Design review of the part shown in the three views and the two pictorial views. Dimensions are in mm from the part's minimum x, y and z. A direction names the side the tool comes from. Round coordinates to 2 decimals unless told otherwise and drop trailing zeros. Order: outer loops, then holes, each group sorted by start corner. A loop starts at its lowest first (then second) coordinate and runs counter-clockwise, first axis right, second up. Notation, with made-up numbers: (18, 72) - (72, 72) arc R4 ccw to (72, 77) - close; hole circle Ø11 at (35.5, -17.5). An arc over 180 degrees is marked (long way). One line per question, with ' | ' between items. Start each with the question number.
Item 1: Tool access review of the marked faces 4, 5, 6 and 7: name each direction out of +Z, -Z, +X, -X, +Y, -Y from which nothing blocks a thin tool from reaching the whole face with its end or side.
Item 2: Add section A-A on y = 6.35. State the section outline as (x, z) points, and give its area (3 significant figures).
Item 3: Draft analysis for pull direction X (two halves, no side actions). For the marked faces 1, 2 and 3, state which applies: +X half, -X half, draft (parallel to the pull), parting line (faces both ways), or undercut.
Item 4: Add section D-D on y = 10.5. State the section outline as (x, z) points.
Item 5: For L1, parallel to X at y = 14.85, z = 19; L2, parallel to Y at x = 5, z = 8; L3, parallel to X at y = 15.1, z = 9, list the stretches that pass through material, from the lowest coordinate up. Write a range as [from, to].
Item 6: Insertion check: pin 1 Ø1 at (y, z) = (13, 14.5) entering from -X; pin 2 Ø8 at (x, z) = (30.5, 22) entering from -Y; pin 3 Ø4 at (y, z) = (1.5, 12.5) entering from +X; pin 4 Ø6 at (x, y) = (52, 14.5) entering from +Z. Each pin has a flat end and moves straight along its axis. Give the tip position at first contact, or say it passes through.
Item 7: Add section C-C on z = 8. State the section outline as (x, y) points.
Item 8: Add section B-B on x = 55. State the section outline as (y, z) points, and give its area (3 significant figures).
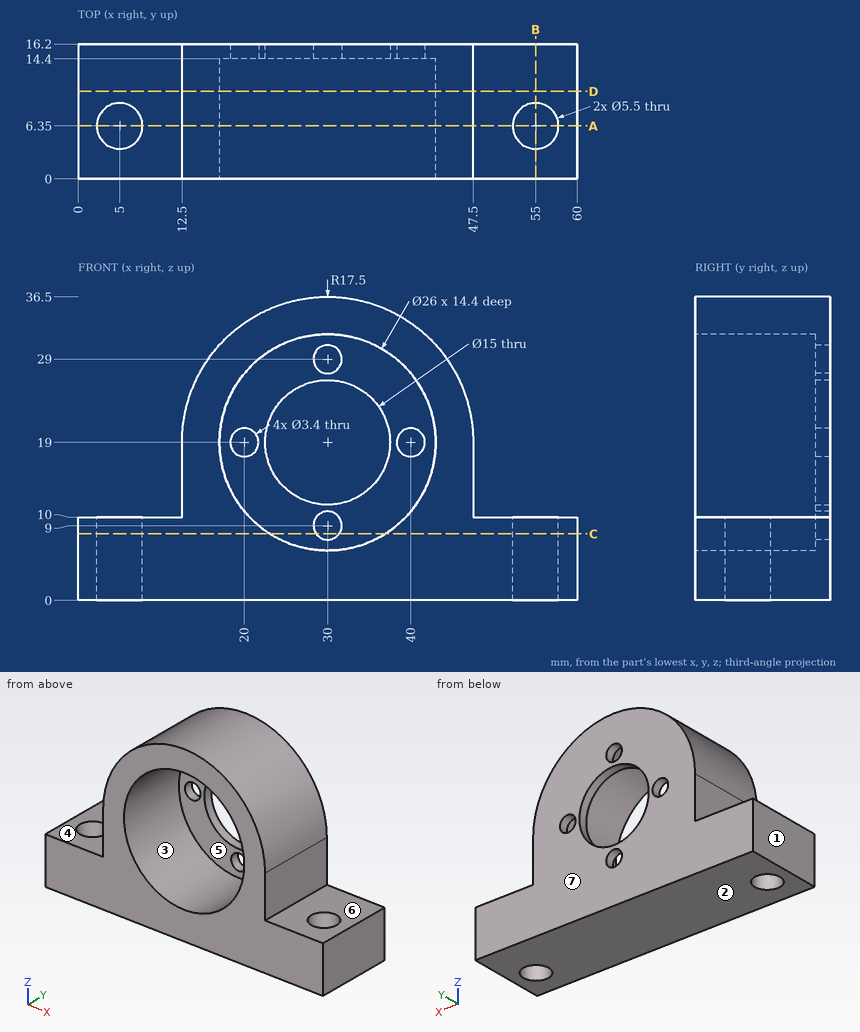
Determined:
1) face 4: +Z, -X, +Y, -Y | face 5: -Y | face 6: +Z, +X, +Y, -Y | face 7: +Z, -Z, +X, -X, +Y
2) outline: (0, 0) - (2.25, 0) - (2.25, 10) - (0, 10) - close; (7.75, 0) - (52.25, 0) - (52.25, 10) - (47.5, 10) - (47.5, 19) arc R17.5 ccw to (12.5, 19) - (12.5, 10) - (7.75, 10) - close; (57.75, 0) - (60, 0) - (60, 10) - (57.75, 10) - close; hole circle Ø26 at (30, 19) | area: 755 mm2
3) face 1: -X half | face 2: draft | face 3: undercut
4) outline: (0, 0) - (60, 0) - (60, 10) - (47.5, 10) - (47.5, 19) arc R17.5 ccw to (12.5, 19) - (12.5, 10) - (0, 10) - close; hole circle Ø26 at (30, 19)
5) L1: [12.5, 18.3], [21.7, 22.5], [37.5, 38.3], [41.7, 47.5] | L2: [0, 3.6], [9.1, 16.2] | L3: [0, 28.3], [31.7, 60]
6) pin 1: x = 12.5 | pin 2: through | pin 3: x = 47.5 | pin 4: z = 10
7) outline: (0, 0) - (23.07, 0) - (23.07, 14.4) - (28.63, 14.4) - (28.63, 16.2) - (0, 16.2) - close; (31.37, 14.4) - (36.93, 14.4) - (36.93, 0) - (60, 0) - (60, 16.2) - (31.37, 16.2) - close; hole circle Ø5.5 at (5, 6.35); hole circle Ø5.5 at (55, 6.35)
8) outline: (0, 0) - (3.6, 0) - (3.6, 10) - (0, 10) - close; (9.1, 0) - (16.2, 0) - (16.2, 10) - (9.1, 10) - close | area: 107 mm2
